Geometry: final body of the model. Coordinates: model frame, mm. Face numbers are marked on the shaded views. A direction names the side the tool comes from. Coordinates: 2 decimals unless noted, no trailing zeros. Write each loop counter-clockwise with the first axis right and the second up, starting at its lowest first coordinate (ties: lowest second). Pieces come first, ordered by that corner, then holes.
from build123d import *


with BuildPart() as part:
    # Schizzo1 → Rivoluzione1 (revolve)
    with BuildSketch(Plane.XY, mode=Mode.PRIVATE) as rivoluzione1_sk:
        with BuildLine():
            Line((0, 0), (-23.453565926, 0))
            ThreePointArc((-23.453565926, 0), (-26.81732667, 1.300660375), (-28.431043289, 4.525954537))
            Line((-28.431043289, 4.525954537), (-29.945842771, 20.431349098))
            ThreePointArc((-29.945842771, 20.431349098), (-29.967481843, 20.999388589), (-29.924504912, 21.566213162))
            Line((-29.924504912, 21.566213162), (-28, 36))
            Line((-28, 36), (-28, 127))
            ThreePointArc((-28, 127), (-28.901772547, 148.408088308), (-18.25, 167))
            Line((-18.25, 167), (-13, 218))
            Line((-13, 218), (-13, 230))
            Line((-13, 230), (-8.5, 230))
            Line((-8.5, 230), (-8.5, 225.5))
            Line((-8.5, 225.5), (-8.5, 217.76899273))
            Line((-8.5, 217.76899273), (-13.947509535, 164.850328678))
            ThreePointArc((-13.947509535, 164.850328678), (-24.422294077, 147.77127274), (-23.5, 127.757161803))
            Line((-23.5, 127.757161803), (-23.5, 35.701321612))
            Line((-23.5, 35.701321612), (-25.463979359, 20.971476422))
            ThreePointArc((-25.463979359, 20.971476422), (-25.468277052, 20.914793964), (-25.466113145, 20.857990015))
            Line((-25.466113145, 20.857990015), (-23.951313663, 4.952595454))
            ThreePointArc((-23.951313663, 4.952595454), (-23.789942001, 4.630066038), (-23.453565926, 4.5))
            Line((-23.453565926, 4.5), (0, 4.5))
            Line((0, 4.5), (0, 0))
        make_face()
    revolve(rivoluzione1_sk.sketch.rotate(Axis((0, 0, 0), (0, 1, 0)), 270), axis=Axis((0, 0, 0), (0, 1, 0)))


solid = part.part
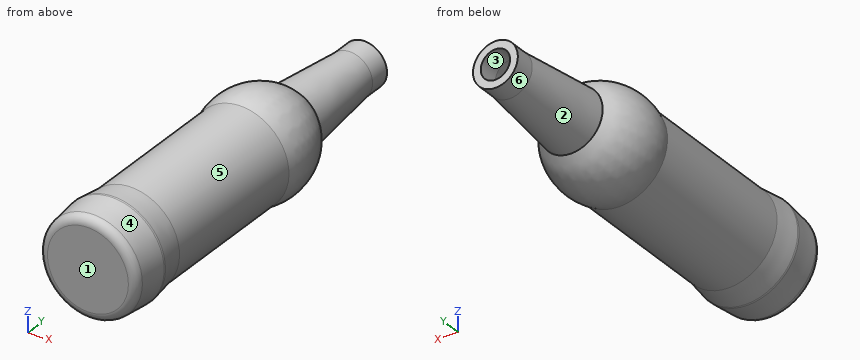
Item 1: Section A-A, the plane y = 46. Output: boundary loops of the cut face in (x, z).
Derived:
outline: circle Ø56 at (0, 0); hole circle Ø47 at (0, 0)
Item 2: Pull-direction query (X, two-part tool) for the marked faces 1, 2 and 3; classes: released by +X, released by -X, zero draft, split by the parting line, or undercut.
Derived:
face 1: zero draft
face 2: split by the parting line
face 3: undercut
Item 3: Set-up query: the marked faces 4, 5 and 6. Return all of +Z, -Z, +X, -X, +Y, -Y with unobstructed straight access to the full face (end or side cutting, diameter ignored); none if empty.
Derived:
face 4: -Y
face 5: none
face 6: +Y
Item 4: Pin query (flat end, axial travel): pin 1 (4 mm diameter, centred on x = 24, y = 120, fed in from +Z); pin 2 (15.5 mm diameter, centred on x = 0, z = 0, fed in from +Y); pin 3 (5 mm diameter, centred on y = 36.5, z = -7.5, fed in from +X). Return the tip coordinate at first contact, or that it passes through.
Derived:
pin 1: stops at z = 17.32
pin 2: stops at y = 4.5
pin 3: stops at x = 27.59
Item 5: Material intervals for probe 1 along X at (y, z) = (118, 0); probe 2 along X at (y, z) = (200, -5); probe 3 along Y at (x, z) = (-13.5, 17.5), sorted ascending.
Derived:
probe 1: x = -28 to -23.5, 23.5 to 28
probe 2: x = -13.99 to -9.04, 9.04 to 13.99
probe 3: y = 0 to 4.5, 154.11 to 162.66
Item 6: Section B-B, the plane y = 194.5. Output: boundary loops of the cut face in (x, z).
Derived:
outline: circle Ø30.84 at (0, 0); hole circle Ø21.79 at (0, 0)
